Can you work these out from the model? Positions are in its coordinate system, mm. Give positions to 0.01 mm unless a question says otherwise; leave off trailing zeros. Order: outer loops, then holes, each group sorted by start corner. A loop starts at its lowest first (then second) coordinate and runs counter-clockwise, first axis right, second up. Notation, with made-up numbers: M 85,-28 L 120,-28 A33 ccw 120,1 Z; hole C 65,-9 d1. An arc over 180 degrees is marked long. Use one line per item in the form item = value. Start each with the question number.
1. I want a section at A-A, the plane y = 1.1. List the corners of the cut face in (x, z) for me, and give its area (3 significant figures).
2. I want a section at C-C, the plane x = 18. List the corners of the cut face in (y, z) for me.
3. I need wall thicknesses on L1, parallel to Z at x = 21, y = 1.4; L2, parallel to X at y = 0.5, z = -42.5; L3, parallel to X at y = 1.45, z = -39.5. Which ranges of each line are inside material? Lowest first, please.
4. I want a section at B-B, the plane x = -20.5. List the corners of the cut face in (y, z) for me, and give its area (3 significant figures).
5. Will these pins go through, and if not, where does the flat tip stop? P1, Ø4, axis at x = 20.5, z = 10.84, coming from the -Y side; P2, Ø1, axis at x = 16.5, y = 1.5, coming from the -Z side.
6. We'd pull the mould along X, two halves only. Please class faces 1 (the face through (-19.013, 0.986, -24.353)), 2 (the face through (-36, 1, 0)), 3 (the face through (17.748, 0.986, -42.675)): +X half, -X half, draft (parallel to the pull), parting line (faces both ways), or undercut.
7. I want a section at D-D, the plane x = -9.5. List the corners of the cut face in (y, z) for me.
```python
from build123d import *

# Parameters (mm, degrees)
SKETCH1_R           = 1.5
BOSS_EXTRUDE1_DEPTH = 2


with BuildPart() as part:
    # Sketch1 → Boss-Extrude1 (new body)
    with BuildSketch(Plane(origin=(0, 0, 0), x_dir=(1, 0, 0), z_dir=(0, 1, 0))):
        Polygon((-36, -30), (-36, 30), (0, 55), (36, 30), (36, -30), align=None)
        with Locations(Location((-20.5, 24.157329938, 0), (0, 0, 270))):
            Circle(SKETCH1_R, mode=Mode.SUBTRACT)
        with Locations(Location((20.5, 24.157329938, 0), (0, 0, 270))):
            Circle(SKETCH1_R, mode=Mode.SUBTRACT)
        with Locations(Location((20.5, -10.842670062, 0), (0, 0, 270))):
            Circle(SKETCH1_R, mode=Mode.SUBTRACT)
        with Locations(Location((-20.5, -10.842670062, 0), (0, 0, 270))):
            Circle(SKETCH1_R, mode=Mode.SUBTRACT)
    extrude(amount=BOSS_EXTRUDE1_DEPTH)


solid = part.part
```
Check result:
q1.outline = M -36,-30 L 0,-55 L 36,-30 L 36,30 L -36,30 Z; hole C -20.5,-24.16 d3; hole C -20.5,10.84 d3; hole C 20.5,-24.16 d3; hole C 20.5,10.84 d3
q1.area = 5,190 mm2
q2.outline = M 0,-42.5 L 2,-42.5 L 2,30 L 0,30 Z
q3.L1 = -40.42 to -25.57, -22.74 to 9.43, 12.26 to 30
q3.L2 = -18 to 18
q3.L3 = -22.32 to 22.32
q4.outline = M 0,-40.76 L 2,-40.76 L 2,-25.66 L 0,-25.66 Z; M 0,-22.66 L 2,-22.66 L 2,9.34 L 0,9.34 Z; M 0,12.34 L 2,12.34 L 2,30 L 0,30 Z
q4.area = 130 mm2
q5.P1 = 0
q5.P2 = -43.89
q6.face_1 = undercut
q6.face_2 = -X half
q6.face_3 = +X half
q7.outline = M 0,-48.4 L 2,-48.4 L 2,30 L 0,30 Z
